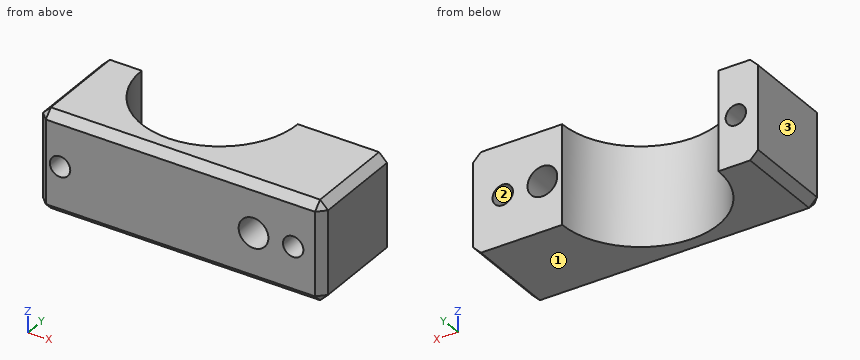
from build123d import *

# Parameters (mm, degrees)
BOSS_EXTRUDE1_DEPTH                 = 31.75
F_5_16_18_TAPPED_HOLE1_D            = 6.5278
F_3_8_0_375_CLEARANCE_DOWEL_HOLE2_D = 9.525
CHAMFER1_SIZE                       = 2.54


with BuildPart() as part:
    # Sketch1 → Boss-Extrude1 (new body)
    with BuildSketch(Plane.XY):
        with BuildLine():
            Line((0, 0), (12.7, 0))
            ThreePointArc((12.7, 0), (37.719, -25.019), (62.738, 0))
            Line((62.738, 0), (91.313, 0))
            Line((91.313, 0), (91.313, -31.496))
            Line((91.313, -31.496), (0, -31.496))
            Line((0, -31.496), (0, 0))
        make_face()
    extrude(amount=BOSS_EXTRUDE1_DEPTH)

    # 5/16-18 Tapped Hole1 (through all)
    with Locations(Plane(origin=(0, -31.496, 0), x_dir=(-1, 0, 0), z_dir=(0, -1, 0))):
        with Locations((-7.1247, -15.875), (-81.788, -15.875)):
            Hole(F_5_16_18_TAPPED_HOLE1_D / 2)

    # 3/8 (0.375) Clearance Dowel Hole2 (through all)
    with Locations(Plane(origin=(0, -31.496, 0), x_dir=(-1, 0, 0), z_dir=(0, -1, 0))):
        with Locations((-69.088, -15.875)):
            Hole(F_3_8_0_375_CLEARANCE_DOWEL_HOLE2_D / 2)

    # Chamfer1
    chamfer1_edges = [part.edges().sort_by_distance(p)[0] for p in [
        (91.313, -15.748, 31.75),
        (91.313, -31.496, 15.875),
        (0, -31.496, 15.875),
        (0, -15.748, 31.75),
        (45.6565, -31.496, 31.75),
        (91.313, -15.748, 0),
        (45.6565, -31.496, 0),
        (0, -15.748, 0),
    ]]
    chamfer(chamfer1_edges, length=CHAMFER1_SIZE)


solid = part.part
Work out the finished part from the listing and answer in its coordinate system (mm). Face numbers are marked on the shaded views. Give positions to 0.01 mm unless a question says otherwise; leave off trailing zeros. Order: outer loops, then holes, each group sorted by start corner. A loop starts at its lowest first (then second) coordinate and runs counter-clockwise, first axis right, second up. Notation, with made-up numbers: M 82,-8 L 93,-8 A24 cw 93,21 Z; hole C 71.25,4 d5. An arc over 180 degrees is marked long. Return JSON: item names as keys, results as strings.
Q1. Find section B-B, the plane x = 83. Write down the section's boundary in (y, z).
Answer below:
{"outline": "M -31.5,2.54 L -28.96,0 L 0,0 L 0,12.84 L -31.5,12.84 Z; M -31.5,18.91 L 0,18.91 L 0,31.75 L -28.96,31.75 L -31.5,29.21 Z"}
Q2. The mould has two halves that part along Z. Classify the marked faces 1, 2 and 3: pulls with the +Z half, pulls with the -Z half, needs draft (parallel to the pull), parting line crosses it, or undercut.
Answer below:
{"face 1": "pulls with the -Z half", "face 2": "undercut", "face 3": "needs draft"}
Q3. Find section D-D, the plane z = 27. Write down the section's boundary in (x, y).
Answer below:
{"outline": "M 0,-28.96 L 2.54,-31.5 L 88.77,-31.5 L 91.31,-28.96 L 91.31,0 L 62.74,0 A25.02 cw 12.7,0 L 0,0 Z"}
Q4. This flat-tipped pin is pushed along its axis until it touches: pin 1 (1 mm diameter, centred on x = 41.5, z = 7, fed in from +Y). Where does it stop, or does it pass through?
Answer below:
{"pin 1": "stops at y = -24.65"}
Q5. Find the intervals of material crossed by line 1 along X through (y, z) = (-18, 13.5); line 2 along X through (y, z) = (-15, 13); line 3 along X through (y, z) = (-23, 12.5), in increasing order. Write a range as [from, to].
Answer below:
{"line 1": "x = [0, 4.89], [9.36, 20.34], [55.1, 64.96], [73.22, 79.55], [84.03, 91.31]", "line 2": "x = [0, 5.58], [8.67, 17.7], [57.74, 65.29], [72.88, 80.24], [83.33, 91.31]", "line 3": "x = [0, 27.87], [47.57, 65.73], [72.45, 91.31]"}
Q6. Find section A-A, the plane y = -20. State how many separate pieces and enclosed holes the cut face has, and give its area (3 significant figures).
Answer below:
{"separate pieces": "2", "enclosed holes": "3", "area": "1,790 mm^2"}
